Read the model definition and answer for the solid it produces. Units are mm, in the model's axes. A direction names the side the tool comes from. Coordinates: 2 decimals unless noted, no trailing zeros. Order: outer loops, then holes, each group sorted by start corner. A loop starts at its lowest first (then second) coordinate and runs counter-clockwise, first axis right, second up. Notation, with made-up numbers: M 2,-36.5 L 46,-36.5 A14 cw 46,-14.5 Z; hole C -18.75,-4 d10. An arc over 180 degrees is marked long. Use a Markdown table: item, result. Add a question column.
1) Each of these flat-tipped pins is pushed along its axis until it touches: pin 1 Ø8 at (x, z) = (33.5, 305.5) entering from +Y; pin 2 Ø3 at (y, z) = (-42.5, 153) entering from -X; pin 3 Ø1.5 at (x, y) = (38, -30.5) entering from +Z; pin 4 Ø8 at (x, z) = (45, 75) entering from +Y. Where does it stop, or does it pass through?
2) For faces 1 (the face through (-8, -10, 406.4)), 2 (the face through (27, -50, 101.6)), determine the directions among +Z, -Z, +X, -X, +Y, -Y from which every point of the face is accessible in a straight line to the end or side of a thin tool.
3) The mould has two halves that part along Y. Classify faces 3 (the face through (14.6, -59.5, 76.2)), 4 (the face through (6.48, 18.39, 367.77)), 5 (the face through (-23.355, -17.908, 266.522)): released by +Y, released by -Y, zero draft, split by the parting line, or undercut.
4) Find section A-A on z = 95.5. Write down the section's boundary in (x, y), plus the area to 3 significant figures.
5) Find the intervals of material crossed by probe 1 along X at (y, z) = (12.5, 344); probe 2 along Z at (x, y) = (-14, -21.5); probe 3 along Z at (x, y) = (26, 16.5), in increasing order. Write a range as [from, to].
from build123d import *

# Parameters (mm, degrees)
F0_R      = 79.5450036975
F1_DEPTH  = 25.4
F2_R      = 73.7515149203
F3_DEPTH  = 25.4
F4_R      = 67.2732126862
F5_DEPTH  = 25.4
F6_R      = 61.109227751
F7_DEPTH  = 25.4
F8_R      = 56.3027484013
F9_DEPTH  = 25.4
F10_R     = 51.3446313858
F11_DEPTH = 25.4
F12_R     = 46.7578066383
F13_DEPTH = 25.4
F14_R     = 42.0901979961
F15_DEPTH = 25.4
F16_R     = 37.5067154874
F17_DEPTH = 25.4
F18_R     = 33.3373265509
F19_DEPTH = 25.4
F20_R     = 29.4310817061
F21_DEPTH = 25.4
F22_R     = 26.0855959035
F23_DEPTH = 25.4
F24_R     = 22.3736631593
F25_DEPTH = 25.4
F26_R     = 3.4212934719
F26_R_2   = 3.8149535716
F26_R_3   = 4.641761037
F26_R_4   = 3.4439254553
F26_R_5   = 3.753363135
F26_R_6   = 6.9663604667
F27_DEPTH = 76.2


with BuildPart() as f1:
    # F0 (on Top) → F1 (new body)
    with BuildSketch(Plane.XY):
        Circle(F0_R)
    extrude(amount=F1_DEPTH)

    # F2 (on face) → F3 (join)
    with BuildSketch(Plane.XY.offset(25.4)):
        Circle(F2_R)
    extrude(amount=F3_DEPTH)

    # F4 (on face) → F5 (join)
    with BuildSketch(Plane.XY.offset(50.8)):
        Circle(F4_R)
    extrude(amount=F5_DEPTH)

    # F6 (on face) → F7 (join)
    with BuildSketch(Plane.XY.offset(76.2)):
        Circle(F6_R)
    extrude(amount=F7_DEPTH)

    # F8 (on face) → F9 (join)
    with BuildSketch(Plane.XY.offset(101.6)):
        Circle(F8_R)
    extrude(amount=F9_DEPTH)

    # F10 (on face) → F11 (join)
    with BuildSketch(Plane.XY.offset(127)):
        Circle(F10_R)
    extrude(amount=F11_DEPTH)

    # F12 (on face) → F13 (join)
    with BuildSketch(Plane.XY.offset(152.4)):
        Circle(F12_R)
    extrude(amount=F13_DEPTH)

    # F14 (on face) → F15 (join)
    with BuildSketch(Plane.XY.offset(177.8)):
        Circle(F14_R)
    extrude(amount=F15_DEPTH)

    # F16 (on face) → F17 (join)
    with BuildSketch(Plane.XY.offset(203.2)):
        Circle(F16_R)
    extrude(amount=F17_DEPTH)

    # F18 (on face) → F19 (join)
    with BuildSketch(Plane.XY.offset(228.6)):
        Circle(F18_R)
    extrude(amount=F19_DEPTH)

    # F20 (on face) → F21 (join)
    with BuildSketch(Plane.XY.offset(254)):
        Circle(F20_R)
    extrude(amount=F21_DEPTH)

    # F22 (on face) → F23 (join)
    with BuildSketch(Plane.XY.offset(279.4)):
        Circle(F22_R)
    extrude(amount=F23_DEPTH)

    # F24 (on face) → F25 (join)
    with BuildSketch(Plane.XY.offset(304.8)):
        Circle(F24_R)
    extrude(amount=F25_DEPTH)

    # F26 (on face) → F27 (join)
    with BuildSketch(Plane.XY.offset(330.2)):
        with Locations((-8.4204990417, 12.5169595703)):
            Circle(F26_R)
        with BuildLine():
            ThreePointArc((-12.8764627366, 4.7200013898), (-16.9768846981, -3.1594538942), (-8.6752507068, 0))
            ThreePointArc((-8.6752507068, 0), (-9.1506984309, 2.071867738), (-10.4819031466, 3.7291487844))
            ThreePointArc((-10.4819031466, 3.7291487844), (-11.7969854067, 3.9398859003), (-12.8764627366, 4.7200013898))
        make_face()
        with BuildLine():
            ThreePointArc((-12.8764627366, 4.7200013898), (-11.7969854067, 3.9398859003), (-10.4819031466, 3.7291487844))
            ThreePointArc((-10.4819031466, 3.7291487844), (-11.6103347479, 4.3909581613), (-12.8764627366, 4.7200013898))
        make_face()
        with BuildLine():
            ThreePointArc((-12.8764627366, 4.7200013898), (-11.6103347479, 4.3909581613), (-10.4819031466, 3.7291487844))
            ThreePointArc((-10.4819031466, 3.7291487844), (-8.5863196556, 4.6415751091), (-7.8176113456, 6.5998514183))
            ThreePointArc((-7.8176113456, 6.5998514183), (-11.6990310984, 9.298268247), (-12.8764627366, 4.7200013898))
        make_face()
        with Locations((-8.4204990417, -10.0135672837)):
            Circle(F26_R_2)
        with Locations((12.289378792, 0)):
            Circle(F26_R_3)
        with Locations((10.69631055, -8.6480807513)):
            Circle(F26_R_4)
        with Locations((0, -10.69631055)):
            Circle(F26_R_5)
        with Locations((2.7309742291, 12.5169595703)):
            Circle(F26_R_6)
    extrude(amount=F27_DEPTH)


solid = f1.part
Check result:
| question | item | result |
|---|---|---|
| 1 | pin 1 | passes through |
| 1 | pin 2 | stops at x = -30.74 |
| 1 | pin 3 | stops at z = 152.4 |
| 1 | pin 4 | stops at y = 53.34 |
| 2 | face 1 | +Z, +X, -X, +Y, -Y |
| 2 | face 2 | +Z |
| 3 | face 3 | zero draft |
| 3 | face 4 | undercut |
| 3 | face 5 | split by the parting line |
| 4 | outline | C 0,0 d122.22 |
| 4 | area | 11,700 mm2 |
| 5 | probe 1 | x = [-11.84, -5], [-4.24, 9.7] |
| 5 | probe 2 | z = [0, 304.8] |
| 5 | probe 3 | z = [0, 254] |
